Could you check a few things on this model? Use its own coordinates, in mm. A direction names the side the tool comes from. Coordinates: 2 decimals unless noted, no trailing zeros. Loops run counter-clockwise (first coordinate to the right, second up) from the corner with the lowest first, then second, coordinate; pieces in that order, holes last. Notation, with made-up numbers: (9, -15.5) - (36, -15.5) arc R15 ccw to (36, -2.5) - close; hole circle Ø3 at (34.5, 88). An arc over 180 degrees is marked (long way). Put each result on its own line as item: value. Start each with the question number.
```python
from build123d import *

# Parameters (mm, degrees)
SKETCH1_R           = 24.765
SKETCH1_R_2         = 20.6375
BOSS_EXTRUDE1_DEPTH = 76.2
SKETCH2_R           = 9.525
CUT_EXTRUDE1_DEPTH  = 76.2
SKETCH3_R           = 13.335
SKETCH3_R_2         = 9.525
BOSS_EXTRUDE2_DEPTH = 25.4
BOSS_EXTRUDE3_START = 3.4
SKETCH4_R           = 13.335
SKETCH4_R_2         = 9.525
BOSS_EXTRUDE3_DEPTH = 3.4


with BuildPart() as part:
    # Sketch1 → Boss-Extrude1 (new body)
    with BuildSketch(Plane.XY):
        with Locations(Location((0, 0, 0), (0, 0, 180))):
            Circle(SKETCH1_R)
        with Locations(Location((0, 0, 0), (0, 0, 180))):
            Circle(SKETCH1_R_2, mode=Mode.SUBTRACT)
    extrude(amount=BOSS_EXTRUDE1_DEPTH)

    # Sketch2 → Cut-Extrude1 (cut)
    with BuildSketch(Plane(origin=(0, 0, 0), x_dir=(0, 0, -1), z_dir=(1, 0, 0))):
        with Locations(Location((-38.1, 0, 0), (0, 0, 180))):
            Circle(SKETCH2_R)
    extrude(amount=-CUT_EXTRUDE1_DEPTH, mode=Mode.SUBTRACT)

    # Sketch3 → Boss-Extrude2 (add)
    with BuildSketch(Plane(origin=(-24.13, 0, 0), x_dir=(0, 0, -1), z_dir=(1, 0, 0))):
        with Locations((-38.1, 0)):
            Circle(SKETCH3_R)
        with Locations((-38.1, 0)):
            Circle(SKETCH3_R_2, mode=Mode.SUBTRACT)
    extrude(amount=-BOSS_EXTRUDE2_DEPTH)

    # Sketch4 → Boss-Extrude3 (add)
    with BuildSketch(Plane(origin=(-24.13, 0, 0), x_dir=(0, 0, -1), z_dir=(1, 0, 0)).offset(BOSS_EXTRUDE3_START)):
        with Locations((-38.1, 0)):
            Circle(SKETCH4_R)
        with Locations((-38.1, 0)):
            Circle(SKETCH4_R_2, mode=Mode.SUBTRACT)
    extrude(amount=-BOSS_EXTRUDE3_DEPTH)


solid = part.part
```
(1) If we mould it in two halves opening along X, with no side actions, what happens to faces 1 (the flat face through (6, -20, 76.2)), 2 (the cylindrical face through (20.618, -0.907, 37.567)), 3 (the cylindrical face through (24.74, -1.09, 37.57))? For each: pulls with the +X half, pulls with the -X half, needs draft (parallel to the pull), parting line crosses it, or undercut.
(2) I want a section at A-A on x = 0. List the corners of the cut face in (y, z) for me (1 decimal), and give its area (3 significant figures).
(3) I need wall thicknesses on L1, parallel to Y at x = -34, z = 38.1 (3 decimals); L2, parallel to Y at x = 0, z = 38 (1 decimal); L3, parallel to X at y = -14.5, z = 54.5. Which ranges of each line are inside material? Lowest first, please. Write a range as [from, to].
(4) I want a section at B-B on y = 16. List the corners of the cut face in (x, z) for me.
(5) For pin 1 Ø6 at (y, z) = (18, 49.5) entering from -X; pin 2 Ø5 at (y, z) = (-5, 61) entering from -X; pin 3 Ø4 at (y, z) = (-17.5, 47.5) entering from -X; pin 4 Ø12 at (x, y) = (8, 11.5) entering from +Z, each with a flat end and sliding along its axis, tell me the tip position at first contact or that it passes through.
(6) Which directions (+Z, -Z, +X, -X, +Y, -Y) give clear straight access to the entire face, cutting with the end or side of a thin tool? Please do faces 4 (the cylindrical face through (-33.7, 9.504, 37.472)), 5 (the flat face through (6, -20, 0)).
(7) I want a section at C-C on z = 16. List the corners of the cut face in (x, y) for me (1 decimal).
Answer sheet:
1. face 1: needs draft
1. face 2: undercut
1. face 3: parting line crosses it
2. outline: (-24.8, 0) - (-20.6, 0) - (-20.6, 76.2) - (-24.8, 76.2) - close; (20.6, 0) - (24.8, 0) - (24.8, 76.2) - (20.6, 76.2) - close
2. area: 629 mm^2
3. L1: y = [-13.335, -9.525], [9.525, 13.335]
3. L2: y = [-24.8, -20.6], [20.6, 24.8]
3. L3: x = [-20.08, -14.69], [14.69, 20.08]
4. outline: (-18.9, 0) - (-13.03, 0) - (-13.03, 76.2) - (-18.9, 76.2) - close; (13.03, 0) - (18.9, 0) - (18.9, 76.2) - (13.03, 76.2) - close
5. pin 1: stops at x = -19.71
5. pin 2: stops at x = -24.64
5. pin 3: stops at x = -19.31
5. pin 4: passes through
6. face 4: -X
6. face 5: -Z, +X, -X, +Y, -Y
7. outline: circle Ø49.5 at (0, 0); hole circle Ø41.3 at (0, 0)
